Verification items for this drawing (mm, ordinates from the low corner). Round coordinates to 2 decimals unless told otherwise and drop trailing zeros. Order: outer loops, then holes, each group sorted by start corner. A loop starts at its lowest first (then second) coordinate and runs counter-clockwise, first axis right, second up.
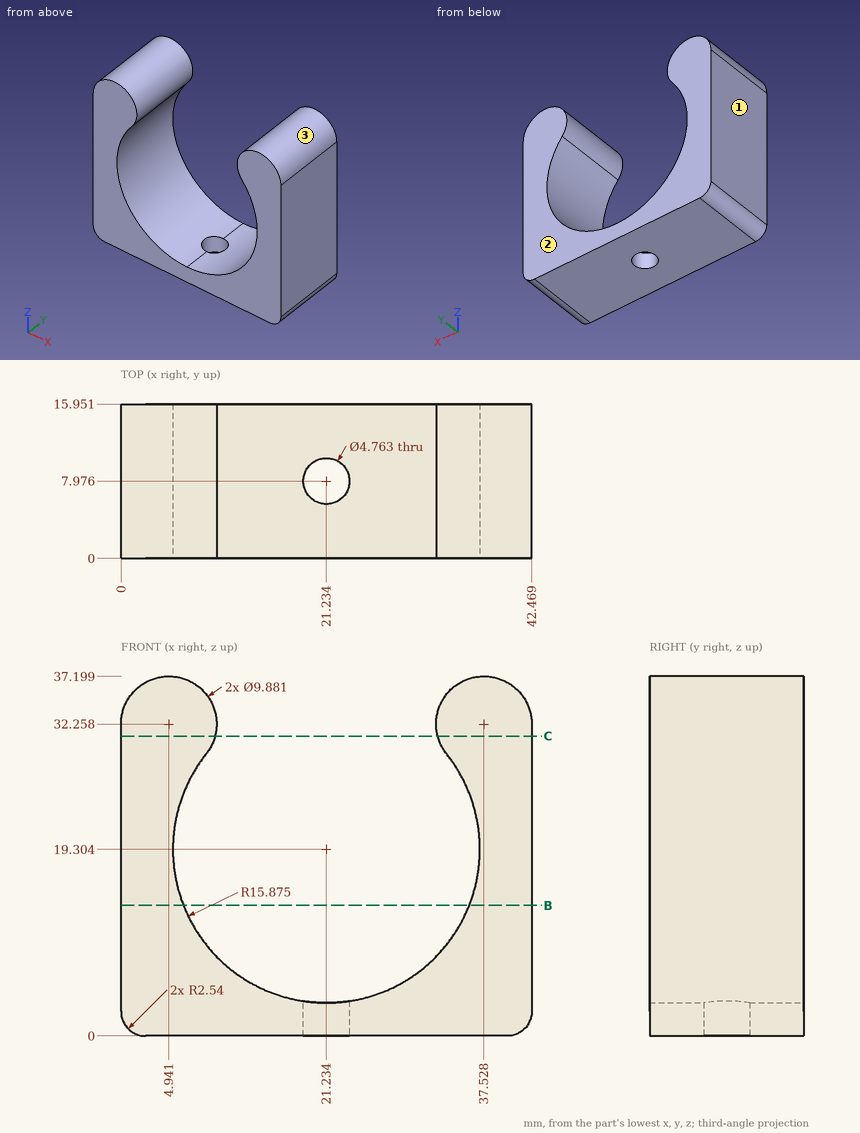
Item 1: Sectioned sample at C-C (z = 31). Record the cut outline in (x, y).
Answer:
outline: (0, 0) - (9.72, 0) - (9.72, 15.95) - (0, 15.95) - close; (32.75, 0) - (42.47, 0) - (42.47, 15.95) - (32.75, 15.95) - close
Item 2: Sectioned sample at B-B (z = 13.5). Record the cut outline in (x, y).
Answer:
outline: (0, 0) - (6.46, 0) - (6.46, 15.95) - (0, 15.95) - close; (36.01, 0) - (42.47, 0) - (42.47, 15.95) - (36.01, 15.95) - close
Item 3: Go/stop test with flat-tipped pins: P1, Ø1, axis at x = 9, y = 9, coming from the +Z side (1 decimal); P2, Ø6, axis at x = 21.23, y = 7.98, coming from the +Z side. Record where each tip stops, or that it passes through.
Answer:
P1: stops at z = 35.7
P2: stops at z = 3.72
Item 4: Scan lines: line 1 along Z through (x, y) = (34.5, 15) (1 decimal); line 2 along X through (y, z) = (6.5, 27.5); line 3 along X through (y, z) = (9.25, 28) (1 decimal). Record each from-to range of solid material in increasing order.
Answer:
line 1: z = 0 to 10.6, 28 to 36.2
line 2: x = 0 to 7.64, 34.83 to 42.47
line 3: x = 0 to 8, 34.5 to 42.5
Item 5: Release check for a two-part mould opening along X. For the marked faces 1, 2 and 3 record: released by +X, released by -X, zero draft, split by the parting line, or undercut.
Answer:
face 1: released by -X
face 2: zero draft
face 3: undercut
